Model file for the job. Use its own axes, mm. Face numbers are marked on the shaded views. A direction names the side the tool comes from. Coordinates: 2 decimals unless noted, no trailing zeros. Write each loop counter-clockwise with the first axis right and the second up, starting at its lowest first coordinate (ties: lowest second). Pieces come first, ordered by that corner, then holes. Notation, with made-up numbers: M 40.25,48.5 L 70.25,48.5 A20 ccw 70.25,53.5 Z; hole C -13,87 d8. An arc over 180 degrees is marked long. Answer in a Markdown table with one row per item. Add a question column.
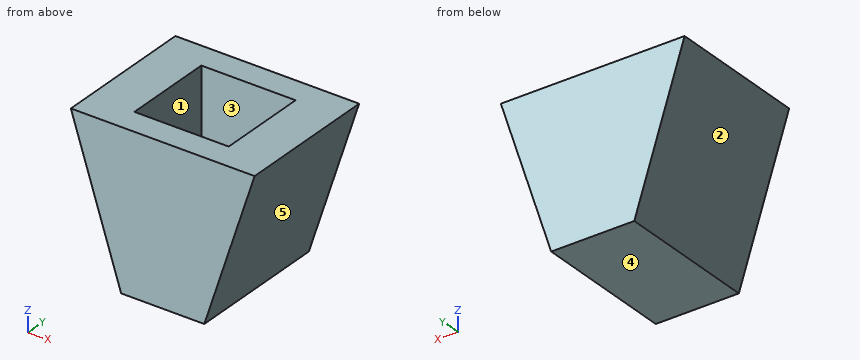
```python
from build123d import *

# Parameters (mm, degrees)
F1_W      = 36.2
F1_H      = 22.2
F2_W      = 12.866667
F2_H      = 22.2
F3_FACE_W = 36.2
F3_FACE_H = 22.2
F4_DEPTH  = 12
F5_W      = 14.6
F5_H      = 14.2
F6_DEPTH  = 32


with BuildPart() as f3:
    # F1 (on offset) → F3 section 0
    with BuildSketch(Plane.XY.offset(36.125)):
        with Locations((0, -11.1)):
            Rectangle(F1_W, F1_H)
    # F2 (on Top) → F3 section 1
    with BuildSketch(Plane.XY):
        with Locations((-3.3e-05, -11.1)):
            Rectangle(F2_W, F2_H)
    loft()

    # F3_face (on face) → F4 (cut)
    with BuildSketch(Plane(origin=(0, -11.1, 36.125), x_dir=(1, 0, 0), z_dir=(0, 0, 1))):
        Rectangle(F3_FACE_W, F3_FACE_H)
    extrude(amount=-F4_DEPTH, mode=Mode.SUBTRACT)

    # F5 (on offset) → F6 (cut)
    with BuildSketch(Plane.XY.offset(36.125)):
        with Locations((0, -11.1)):
            Rectangle(F5_W, F5_H)
    extrude(amount=-F6_DEPTH, mode=Mode.SUBTRACT)


solid = f3.part
```
1) Which spindle directions (+Z, -Z, +X, -X, +Y, -Y) get a long thin tool onto all of the face, cutting with end or side? Do the marked faces 1 and 2. Say none if no direction does.
2) Slice it at A-A (y = -11). Give the cut face in (x, z) (3 decimals), then the cut area to 3 significant figures.
3) Two-plate mould, pull along X, no slides. Class the marked faces 3, 4 and 5: released by +X, released by -X, zero draft, split by the parting line, or undercut.
4) Flat gauge pins, fed straight in: pin 1 Ø10 at (y, z) = (-4.5, 19) entering from +X; pin 2 Ø1 at (y, z) = (-16, 14.5) entering from -X; pin 3 Ø10 at (y, z) = (-9, 17) entering from +X. Where does each tip first touch, or does it go through?
5) Slice it at B-B (y = -19.5). Give the cut face in (x, z) (3 decimals).
6) Drill centre lines: probe 1 along Y at (x, z) = (-4.25, 8.5); probe 2 along X at (y, z) = (-17.5, 11); probe 3 along Z at (x, y) = (4.5, -11.75) (3 decimals). Where is each one in solid material? Low to high.
Ans:
| question | item | result |
|---|---|---|
| 1 | face 1 | +Z |
| 1 | face 2 | -Z, -X, +Y, -Y |
| 2 | outline | M -14.225,24.125 L -6.433,0 L 6.433,0 L 14.225,24.125 L 7.3,24.125 L 7.3,4.125 L -7.3,4.125 L -7.3,24.125 Z |
| 2 | area | 206 mm2 |
| 3 | face 3 | undercut |
| 3 | face 4 | zero draft |
| 3 | face 5 | released by +X |
| 4 | pin 1 | stops at x = 14.18 |
| 4 | pin 2 | stops at x = -11.28 |
| 4 | pin 3 | stops at x = 13.54 |
| 5 | outline | M -14.225,24.125 L -6.433,0 L 6.433,0 L 14.225,24.125 Z |
| 6 | probe 1 | y = -22.2 to -18.2, -4 to 0 |
| 6 | probe 2 | x = -9.99 to -7.3, 7.3 to 9.99 |
| 6 | probe 3 | z = 0 to 4.125 |
